Autodesk Inventor part; units mm, degrees
ref_plane "YZ Plane" through (0, 0, 0) normal (1, 0, 0) x (0, 1, 0)
ref_plane "XZ Plane" through (0, 0, 0) normal (0, 1, 0) x (-1, 0, 0)
ref_plane "XY Plane" through (0, 0, 0) normal (0, 0, 1) x (1, 0, 0)
sketch "Sketch1" plane through (0, 0, 0) normal (1, 0, 0) x (0, 1, 0)
  line L0 (4.25, 0) -> (4.25, -3.75)
  line L1 (0, -2.75) -> (0, 0)
  line L2 (4.75, -2.75) -> (4.75, 0)
  line L3 (4.75, 0) -> (4.25, 0)
  line L4 (4.25, 0) -> (4.25, -2.75)
  line L5 (6.75, -2.75) -> (6.75, -3.75)
  line L6 (6.75, -3.75) -> (4.25, -3.75)
  line L7 (4.75, -2.75) -> (6.75, -2.75)
  point P0 (4.1, 0)
  dimension "d3" = 2.5
  dimension "d4" = 1
  dimension "d5" = 2.75
  dimension "d6" = 4.75
  dimension "d8" = 4.25
revolve "Revolution1" add sketch "Sketch1" angle 360 about axis through (0, 0, -2.75) along (0, 0, 1)
properties part number "Ø10-Ø8Prop"
Read the model definition and answer for the solid it produces. Units are mm, in the model's axes. A direction names the side the tool comes from. Round coordinates to 2 decimals unless told otherwise and drop trailing zeros. Loops run counter-clockwise (first coordinate to the right, second up) from the corner with the lowest first, then second, coordinate; pieces in that order, holes last.
Q1. Section D-D on z = -2.05 is taken. Write down the section's boundary in (x, y).
Q2. Section A-A on x = 0 is taken. Write down the section's boundary in (y, z).
Q3. Which of the six approach directions +Z, -Z, +X, -X, +Y, -Y give full straight-line access (tool end or side, diameter ignored) to faces 1 (the face through (-5, 1, -2.75)), 2 (the face through (-0.1, 4.4, -3.75))?
Q4. Determine the mould class of faces 3 (the face through (3.584, 2.285, -1.901)), 4 (the face through (2, -4, 0)), 5 (the face through (4.214, 2.192, -1.356)) for opening direction X: released by +X, released by -X, zero draft, split by the parting line, or undercut.
Q5. Each of these flat-tipped pins is pushed along its axis until it touches: pin 1 (2 mm diameter, centred on x = 4.5, y = 4.5, fed in from +Z); pin 2 (2 mm diameter, centred on x = -3.5, z = -1.5, fed in from -Y). Where does it stop, or does it pass through?
Q6. Consider probe 1 along X at (y, z) = (0, -3.15); probe 2 along Y at (x, z) = (0, -2.3). Determine where each line is inside the solid, lowest interval first.
Q7. Section C-C on x = -4.5 is taken. Write down the section's boundary in (y, z), and give its area (3 significant figures).
Output:
1. outline: circle Ø9.5 at (0, 0); hole circle Ø8.5 at (0, 0)
2. outline: (-6.75, -3.75) - (-4.25, -3.75) - (-4.25, 0) - (-4.75, 0) - (-4.75, -2.75) - (-6.75, -2.75) - close; (4.25, -3.75) - (6.75, -3.75) - (6.75, -2.75) - (4.75, -2.75) - (4.75, 0) - (4.25, 0) - close
3. face 1: +Z
3. face 2: -Z, +X, -X, +Y, -Y
4. face 3: undercut
4. face 4: zero draft
4. face 5: split by the parting line
5. pin 1: stops at z = -2.75
5. pin 2: stops at y = -4.04
6. probe 1: x = -6.75 to -4.25, 4.25 to 6.75
6. probe 2: y = -4.75 to -4.25, 4.25 to 4.75
7. outline: (-5.03, -3.75) - (5.03, -3.75) - (5.03, -2.75) - (1.52, -2.75) - (1.52, 0) - (-1.52, 0) - (-1.52, -2.75) - (-5.03, -2.75) - close
7. area: 18.4 mm2
